Check sheet for the modelled part. Datum: model origin and axes. Units: mm. A direction names the side the tool comes from. Give positions to 0.01 mm unless a question says otherwise; leave off trailing zeros. Loops run counter-clockwise (first coordinate to the right, second up) from the corner with the lowest first, then second, coordinate; pieces in that order, holes last. Notation, with made-up numbers: M -27,44 L 5,44 A23 cw 5,80 Z; hole C -38,-10.75 d2. An arc over 180 degrees is marked long. Use one line per item in the form item = value.
from build123d import *

# Parameters (mm, degrees)
ESQUISSE1_W             = 42
ESQUISSE1_H             = 42
BOSS_EXTRU_1_DEPTH      = 32.5
CHANFREIN1_SIZE         = 5
CHANFREIN1_SIZE2        = 5.958767963
CHANFREIN1_PART_2_SIZE  = 5
CHANFREIN1_PART_2_SIZE2 = 5.958767963
CHANFREIN1_PART_3_SIZE  = 5
CHANFREIN1_PART_3_SIZE2 = 5.958767963
CHANFREIN1_PART_4_SIZE  = 5
CHANFREIN1_PART_4_SIZE2 = 5.958767963
ESQUISSE2_R             = 11
ESQUISSE2_R_2           = 4.5
BOSS_EXTRU_2_DEPTH      = 1.5
ESQUISSE3_R             = 2.5
BOSS_EXTRU_3_DEPTH      = 20
BOSS_EXTRU_4_DEPTH      = 5.5


with BuildPart() as part:
    # Esquisse1 → Boss.-Extru.1 (new body)
    with BuildSketch(Plane.XY):
        Rectangle(ESQUISSE1_W, ESQUISSE1_H)
    extrude(amount=BOSS_EXTRU_1_DEPTH)

    # Chanfrein1
    chanfrein1_edges = [part.edges().sort_by_distance(p)[0] for p in [
        (21, -21, 16.25),
    ]]
    chanfrein1_side = [part.faces().sort_by_distance(p)[0] for p in [
        (0, -21, 16.25),
    ]]
    chamfer(chanfrein1_edges, length=CHANFREIN1_SIZE, length2=CHANFREIN1_SIZE2, reference=chanfrein1_side[0])

    # Chanfrein1 part 2
    chanfrein1_part_2_edges = [part.edges().sort_by_distance(p)[0] for p in [
        (-21, -21, 16.25),
    ]]
    chanfrein1_part_2_side = [part.faces().sort_by_distance(p)[0] for p in [
        (-21, 0, 16.25),
    ]]
    chamfer(chanfrein1_part_2_edges, length=CHANFREIN1_PART_2_SIZE, length2=CHANFREIN1_PART_2_SIZE2, reference=chanfrein1_part_2_side[0])

    # Chanfrein1 part 3
    chanfrein1_part_3_edges = [part.edges().sort_by_distance(p)[0] for p in [
        (-21, 21, 16.25),
    ]]
    chanfrein1_part_3_side = [part.faces().sort_by_distance(p)[0] for p in [
        (0, 21, 16.25),
    ]]
    chamfer(chanfrein1_part_3_edges, length=CHANFREIN1_PART_3_SIZE, length2=CHANFREIN1_PART_3_SIZE2, reference=chanfrein1_part_3_side[0])

    # Chanfrein1 part 4
    chanfrein1_part_4_edges = [part.edges().sort_by_distance(p)[0] for p in [
        (21, 21, 16.25),
    ]]
    chanfrein1_part_4_side = [part.faces().sort_by_distance(p)[0] for p in [
        (21, 0, 16.25),
    ]]
    chamfer(chanfrein1_part_4_edges, length=CHANFREIN1_PART_4_SIZE, length2=CHANFREIN1_PART_4_SIZE2, reference=chanfrein1_part_4_side[0])

    # Esquisse2 → Boss.-Extru.2 (add)
    with BuildSketch(Plane.XY.offset(32.5)):
        Circle(ESQUISSE2_R)
        Circle(ESQUISSE2_R_2, mode=Mode.SUBTRACT)
    extrude(amount=BOSS_EXTRU_2_DEPTH)

    # Esquisse3 → Boss.-Extru.3 (add)
    with BuildSketch(Plane.XY.offset(32.5)):
        Circle(ESQUISSE3_R)
    extrude(amount=BOSS_EXTRU_3_DEPTH)

    # Esquisse4 → Boss.-Extru.4 (add)
    with BuildSketch(Plane(origin=(0, 21, 0), x_dir=(1, 0, 0), z_dir=(0, 1, 0))):
        Polygon((0, 0), (8.25, 0), (8.25, -10), (-8.25, -10), (-8.25, 0), align=None)
    extrude(amount=BOSS_EXTRU_4_DEPTH)


solid = part.part
1) Section check D-D (y = 9.5). Record the cut outline in (x, z), then the cut area to 3 significant figures.
Evaluation:
outline = M -21,0 L 21,0 L 21,32.5 L 5.55,32.5 L 5.55,34 L -5.55,34 L -5.55,32.5 L -21,32.5 Z
area = 1,380 mm^2
2) Release check for a two-part mould opening along X. For faces 4 (the face through (-0.59, 4.46, 33.24)), 5 (the face through (0, -5, 34)), 6 (the face through (-21, -1, 16)), 7 (the face through (18.535, -17.979, 16.022)) record: pulls with the +X half, pulls with the -X half, needs draft (parallel to the pull), parting line crosses it, or undercut.
Evaluation:
face_4 = undercut
face_5 = needs draft
face_6 = pulls with the -X half
face_7 = pulls with the +X half
3) Depth check by flat-ended pin: pin 1 Ø3 at (y, z) = (23.5, 6.5) entering from +X; pin 2 Ø2 at (y, z) = (1, 40) entering from +X; pin 3 Ø4.5 at (y, z) = (23, 4.5) entering from -X. Enter the tip coordinate at first touch or a pass-through.
Evaluation:
pin_1 = 8.25
pin_2 = 2.5
pin_3 = -16.21
4) Scan lines: line 1 (Y direction, x = 0, z = 33); line 2 (Z direction, x = 5.5, y = 15); line 3 (Y direction, x = -12.5, z = 18). Record each from-to range of solid material in increasing order.
Evaluation:
line_1 = -11 to -4.5, -2.5 to 2.5, 4.5 to 11
line_2 = 0 to 32.5
line_3 = -21 to 21
5) Section check C-C (y = 0). Record the cut outline in (x, z).
Evaluation:
outline = M -21,0 L 21,0 L 21,32.5 L 11,32.5 L 11,34 L 4.5,34 L 4.5,32.5 L 2.5,32.5 L 2.5,52.5 L -2.5,52.5 L -2.5,32.5 L -4.5,32.5 L -4.5,34 L -11,34 L -11,32.5 L -21,32.5 Z
6) Section check B-B (x = 0). Record the cut outline in (y, z), then the cut area to 3 significant figures.
Evaluation:
outline = M -21,0 L 26.5,0 L 26.5,10 L 21,10 L 21,32.5 L 11,32.5 L 11,34 L 4.5,34 L 4.5,32.5 L 2.5,32.5 L 2.5,52.5 L -2.5,52.5 L -2.5,32.5 L -4.5,32.5 L -4.5,34 L -11,34 L -11,32.5 L -21,32.5 Z
area = 1,540 mm^2
7) Section check A-A (z = 6). Record the cut outline in (x, y), then the cut area to 3 significant figures.
Evaluation:
outline = M -21,-16 L -15.04,-21 L 16,-21 L 21,-15.04 L 21,16 L 15.04,21 L 8.25,21 L 8.25,26.5 L -8.25,26.5 L -8.25,21 L -16,21 L -21,15.04 Z
area = 1,800 mm^2
8) Set-up check for faces 1 (the face through (-18.535, 17.979, 16.022)), 2 (the face through (-0.54, -2.44, 42.36)), 3 (the face through (8.25, 24, 5)): record each of +Z, -Z, +X, -X, +Y, -Y from which the full face is reachable in a straight line by a thin tool's end or side.
Evaluation:
face_1 = +Z, -Z, -X, +Y
face_2 = +Z
face_3 = +Z, -Z, +X, +Y
